The listing builds one solid part. Answer for the finished solid, in the listing's coordinates (mm). A direction names the side the tool comes from. Round coordinates to 2 decimals unless told otherwise and drop trailing zeros. Loops run counter-clockwise (first coordinate to the right, second up) from the corner with the lowest first, then second, coordinate; pieces in that order, holes last. Notation, with made-up numbers: M 71.25,85.25 L 88.25,85.25 A10 ccw 88.25,92.25 Z; hole C 62.5,-37.75 d11. An arc over 180 degrees is marked long. Put each result on its own line as item: value. Start each with the question number.
(1) Which of the six approach directions +Z, -Z, +X, -X, +Y, -Y give full straight-line access (tool end or side, diameter ignored) to faces 1 (the face through (-14, 4, 3)), 2 (the face through (0, -27, 19)), 3 (the face through (-7.5, -1, 21))?
(2) Straight lines are drawn through the part: line 1 (Y direction, x = 0, z = 23.3); line 2 (X direction, y = -38, z = 21.2); line 3 (X direction, y = 4, z = 23.5). For each, find the intervals that lie inside material, in ascending order.
(3) Section B-B, the plane z = 6.75 is taken. Determine the outline of the cut face in (x, y).
(4) Section A-A, the plane x = 0 is taken. Determine the outline of the cut face in (y, z).
(5) Flat-ended cylindrical pins translate along their axes: P1, Ø12, axis at x = 13, y = -8, coming from the -Z side; P2, Ø4, axis at x = 16, z = 9, coming from the -Y side; P3, Ø10, axis at x = -15.5, z = 14.5, coming from the -Y side; P4, Ø3, axis at x = -0.5, z = 22.5, coming from the +Y side. Find the tip coordinate at first contact, or state that the pin passes through.
(6) Determine the mould class of faces 4 (the face through (20, -13, 20)), 5 (the face through (0, -24, 25)), 6 (the face through (-0.37, -39.66, 21.96)) for opening direction X: released by +X, released by -X, zero draft, split by the parting line, or undercut.
(7) Section C-C, the plane z = 23.75 is taken. Determine the outline of the cut face in (x, y).
(8) Section D-D, the plane y = -25 is taken. Determine the outline of the cut face in (x, z).
```python
from build123d import *

# Parameters (mm, degrees)
BOX017_W          = 12.5
BOX017_H          = 7.5
BOX017_DEPTH      = 22
BOX020_W          = 12.5
BOX020_H          = 7.5
BOX020_DEPTH      = 22
CYLINDER001_R     = 1.7
CYLINDER001_DEPTH = 30
BOX019_W          = 15
BOX019_H          = 70
BOX019_DEPTH      = 6
BOX018_W          = 40
BOX018_H          = 51
BOX018_DEPTH      = 6


with BuildPart() as cube016:
    # Box017 → Box017 (new body)
    with BuildSketch(Plane(origin=(7.5, 0, 3), x_dir=(1, 0, 0), z_dir=(0, 0, 1))):
        with Locations((6.25, 3.75)):
            Rectangle(BOX017_W, BOX017_H)
    extrude(amount=BOX017_DEPTH)


with BuildPart() as cube019:
    # Box020 → Box020 (new body)
    with BuildSketch(Plane(origin=(-20, 0, 3), x_dir=(1, 0, 0), z_dir=(0, 0, 1))):
        with Locations((6.25, 3.75)):
            Rectangle(BOX020_W, BOX020_H)
    extrude(amount=BOX020_DEPTH)


with BuildPart() as cylinder001:
    # Cylinder001 → Cylinder001 (new body)
    with BuildSketch(Plane(origin=(0, 7, 0), x_dir=(1, 0, 0), z_dir=(0, 0, 1))):
        Circle(CYLINDER001_R)
    extrude(amount=CYLINDER001_DEPTH)


with BuildPart() as cube018:
    # Box019 → Box019 (new body)
    with BuildSketch(Plane(origin=(12.5, 22, 20), x_dir=(1, 0, 0), z_dir=(0, 0, 1))):
        with Locations((7.5, 35)):
            Rectangle(BOX019_W, BOX019_H)
    extrude(amount=BOX019_DEPTH)


with BuildPart() as fusion004004:
    # Box018 → Box018 (new body)
    with BuildSketch(Plane.XY.offset(20)):
        with Locations((20, 25.5)):
            Rectangle(BOX018_W, BOX018_H)
    extrude(amount=BOX018_DEPTH)

    # Cut004013: cut Cube018
    add(cube018.part, mode=Mode.SUBTRACT)


with BuildPart() as fusion004004_1:
    # Cut004013 placement: moved
    add(fusion004004.part.moved(Location((-20, 0, -1))))

    # Cut004014: cut Cylinder001
    add(cylinder001.part, mode=Mode.SUBTRACT)


with BuildPart() as fusion004004_2:
    # Cut004014 placement: moved
    add(fusion004004_1.part.moved(Location((0, -45, 0))))

    # Fusion004004: union Cube016, Cube019
    add(cube016.part)
    add(cube019.part)


solid = fusion004004_2.part
```
Recorded:
1. face 1: -Z, +X, -X, +Y, -Y
1. face 2: -Z, +X, -X, -Y
1. face 3: +Z, -Z, +Y
2. line 1: y = -45 to -39.7, -36.3 to -23
2. line 2: x = -20 to -1.7, 1.7 to 20
2. line 3: x = -20 to -7.5, 7.5 to 20
3. outline: M -20,0 L -7.5,0 L -7.5,7.5 L -20,7.5 Z; M 7.5,0 L 20,0 L 20,7.5 L 7.5,7.5 Z
4. outline: M -45,19 L -39.7,19 L -39.7,25 L -45,25 Z; M -36.3,19 L -23,19 L -23,25 L -36.3,25 Z
5. P1: stops at z = 19
5. P2: stops at y = 0
5. P3: stops at y = -45
5. P4: stops at y = -23
6. face 4: released by +X
6. face 5: zero draft
6. face 6: undercut
7. outline: M -20,-45 L 20,-45 L 20,7.5 L 7.5,7.5 L 7.5,-23 L -7.5,-23 L -7.5,7.5 L -20,7.5 Z; hole C 0,-38 d3.4
8. outline: M -20,19 L 20,19 L 20,25 L -20,25 Z
